Here's how the part is built. I have some questions about the finished solid (model axes, mm). A direction names the side the tool comes from. Coordinates: 2 decimals unless noted, no trailing zeros. Write each loop counter-clockwise with the first axis right and the second up, starting at its lowest first coordinate (ties: lowest second). Pieces come first, ordered by that corner, then holes.
(1) Imagine slicing it at B-B, the plane z = 8. List the corners of the cut face in (x, y) for me.
(2) For pin 1 Ø3 at (x, z) = (5, 7.5) entering from +Y; pin 2 Ø5 at (x, y) = (4, 6) entering from +Z; pin 3 Ø6 at (y, z) = (3.5, -7) entering from +X, each with a flat end and sliding along its axis, tell me the tip position at first contact or that it passes through.
(3) Imagine slicing it at D-D, the plane z = 0. State how many separate pieces and enclosed holes the cut face has, plus the area to 3 significant figures.
(4) Imagine slicing it at C-C, the plane y = 3.75. List the corners of the cut face in (x, z) for me.
(5) Which directions (+Z, -Z, +X, -X, +Y, -Y) give clear straight access to the entire face, cutting with the end or side of a thin tool? Please do faces 5 (the cylindrical face through (-1.464, 10.854, -0.325)), 6 (the cylindrical face through (-4.436, 6.93, 2.307)).
(6) Thinking about a two-plate mould opening in X: for faces 1 (the cylindrical face through (-10.74, 0.99, -2.38)), 2 (the cylindrical face through (0.07, 0.99, -9.5)), 3 (the cylindrical face through (-9.464, 0.986, -0.325)), 4 (the flat face through (-2, 0, 0)), which applies, released by +X, released by -X, zero draft, split by the parting line, or undercut?
(7) Please list where these lines run through material, in increasing order: probe 1 along X at (y, z) = (0.9, 0); probe 2 along Y at (x, z) = (6, 3); probe 3 along X at (y, z) = (1.6, -8).
(8) Imagine slicing it at A-A, the plane x = 8. List the corners of the cut face in (y, z) for me.
```python
from build123d import *

# Parameters (mm, degrees)
SKETCH_1_R               = 11
SKETCH_1_R_2             = 1.5
EXTRUDE_1_DEPTH          = 2
SKETCH_2_R               = 5
EXTRUDE_2_DEPTH          = 10
SKETCH_3_R               = 1.5
CUT_EXTRUDE_1_DEPTH      = 20.646882704
CUT_EXTRUDE_2_DEPTH      = 20.646882704
CUT_EXTRUDE_2_DEPTH_BACK = 20.646882704
SKETCH_5_R               = 1.5


with BuildPart() as part:
    # 草圖1 → 填料-伸長1 (new body)
    with BuildSketch(Plane(origin=(0, 0, 0), x_dir=(1, 0, 0), z_dir=(0, 1, 0))):
        with Locations(Location((0, 0, 0), (0, 0, 270))):
            Circle(SKETCH_1_R)
        with Locations(Location((0, 8, 0), (0, 0, 270))):
            Circle(SKETCH_1_R_2, mode=Mode.SUBTRACT)
        with Locations(Location((8, 0, 0), (0, 0, 270))):
            Circle(SKETCH_1_R_2, mode=Mode.SUBTRACT)
        with Locations(Location((0, -8, 0), (0, 0, 270))):
            Circle(SKETCH_1_R_2, mode=Mode.SUBTRACT)
        with Locations(Location((-8, 0, 0), (0, 0, 270))):
            Circle(SKETCH_1_R_2, mode=Mode.SUBTRACT)
    extrude(amount=EXTRUDE_1_DEPTH)

    # 草圖2 → 填料-伸長2 (add)
    with BuildSketch(Plane(origin=(0, 2, 0), x_dir=(1, 0, 0), z_dir=(0, 1, 0))):
        with Locations(Location((0, 0, 0), (0, 0, 270))):
            Circle(SKETCH_2_R)
    extrude(amount=EXTRUDE_2_DEPTH)

    # 草圖3 → 除料-伸長1 (cut, through all)
    with BuildSketch(Plane(origin=(0, 12, 0), x_dir=(1, 0, 0), z_dir=(0, 1, 0))):
        with Locations(Location((0, 0, 0), (0, 0, 270))):
            Circle(SKETCH_3_R)
    extrude(amount=-CUT_EXTRUDE_1_DEPTH, mode=Mode.SUBTRACT)

    # 草圖5 → 除料-伸長2 (cut, two sides: drawn at the far end of the back side and taken through both)
    with BuildSketch(Plane(origin=(0, 0, 0), x_dir=(-0.7071067811865476, 0, -0.7071067811865476), z_dir=(0.7071067811865476, 0, -0.7071067811865476)).offset(-CUT_EXTRUDE_2_DEPTH_BACK)):
        with Locations((0, 9)):
            Circle(SKETCH_5_R)
    extrude(amount=CUT_EXTRUDE_2_DEPTH + CUT_EXTRUDE_2_DEPTH_BACK, mode=Mode.SUBTRACT)


solid = part.part
```
Recorded:
1. outline: (-7.55, 0) - (-1.5, 0) - (-1.5, 2) - (-7.55, 2) - close; (1.5, 0) - (7.55, 0) - (7.55, 2) - (1.5, 2) - close
2. pin 1: stops at y = 2
2. pin 2: stops at z = 4.77
2. pin 3: stops at x = 10.08
3. separate pieces: 4
3. enclosed holes: 0
3. area: 94.2 mm2
4. outline: circle Ø10 at (0, 0); hole circle Ø3 at (0, 0)
5. face 5: +Y, -Y
5. face 6: +Y
6. face 1: split by the parting line
6. face 2: undercut
6. face 3: undercut
6. face 4: zero draft
7. probe 1: x = -11 to -9.5, -6.5 to -1.5, 1.5 to 6.5, 9.5 to 11
7. probe 2: y = 0 to 2
7. probe 3: x = -7.55 to -1.5, 1.5 to 7.55
8. outline: (0, -7.55) - (2, -7.55) - (2, -1.5) - (0, -1.5) - close; (0, 1.5) - (2, 1.5) - (2, 7.55) - (0, 7.55) - close
